CAD build for the part. Positions are in the model's coordinates, mm. A direction names the side the tool comes from. Give positions to 0.01 mm unless a question says otherwise; leave off trailing zeros. Order: outer loops, then holes, each group sorted by start corner. A loop starts at its lowest first (then second) coordinate and runs counter-clockwise, first axis right, second up. Notation, with made-up numbers: M -29.75,18 L -7.75,18 A24 cw -7.75,52 Z; hole C -17.5,27.25 d2. An arc over 180 degrees is marked long. Put each result on its own line as item: value. Start each with the question number.
1) Cut at B-B (y = 21.5). Write the cut outline in (x, z) (3 decimals).
2) Cut at C-C (x = 14). Write the cut outline in (y, z) (3 decimals).
3) Cut at A-A (x = 37). Write the cut outline in (y, z) (3 decimals), and give its area (3 significant figures).
4) Tool access for faces 4 (the face through (46, -3.048, 2)), 5 (the face through (-7, 71.843, 2)), 6 (the face through (61.722, 83, 2)): list every direction of +Z, -Z, +X, -X, +Y, -Y with a clear straight run to the whole face (end or side of a thin tool).
5) Two-plate mould, pull along X, no slides. Class faces 1 (the face through (64, -3.048, 2)), 2 (the face through (-4.824, 88.582, 1.565)), 3 (the face through (10, -3.048, 2)): released by +X, released by -X, zero draft, split by the parting line, or undercut.
6) Drill centre lines: line 1 (X direction, y = 49, z = 2.4); line 2 (Y direction, x = 3.5, z = 0.4); line 3 (Y direction, x = 14, z = 0.55). Where is each one in solid material? Low to high. Write a range as [from, to].
7) Cut at D-D (z = 0.65). Give the number of separate pieces and of enclosed holes in the cut face, and give its area (3 significant figures).
8) Pin check, flat tips, straight feed: pin 1 (1.6 mm diameter, centred on y = 41, z = 1.5, fed in from +X); pin 2 (1.6 mm diameter, centred on x = 63.5, z = 1, fed in from +Y); pin 3 (0.9 mm diameter, centred on y = -2, z = 1, fed in from +X); pin 4 (3 mm diameter, centred on x = 65.41, y = 75.53, fed in from +Z). Stop position of each tip, or through.
```python
from build123d import *

# Parameters (mm, degrees)
SKETCH1_W           = 12.7
SKETCH1_H           = 3.048
SKETCH1_R           = 1.397
SKETCH1_W_2         = 48.514
SKETCH1_H_2         = 1.8034
BOSS_EXTRUDE1_DEPTH = 3.175
SKETCH6_W           = 48.514
SKETCH6_H           = 3.048
CUT_EXTRUDE2_DEPTH  = 4.175
SKETCH5_R           = 3.6891
SKETCH5_R_2         = 2
BOSS_EXTRUDE3_DEPTH = 3.175


with BuildPart() as part:
    # Sketch1 → Boss-Extrude1 (new body)
    with BuildSketch(Plane.XY):
        with BuildLine():
            Line((38.227, 7.112), (38.227, 0))
            Line((38.227, 0), (38.227, -5.588))
            Line((38.227, -5.588), (59.182, -5.588))
            ThreePointArc((59.182, -5.588), (60.978051224, -4.844051224), (61.722, -3.048))
            Line((61.722, -3.048), (61.722, 86.7664))
            ThreePointArc((61.722, 86.7664), (60.978051224, 88.562451224), (59.182, 89.3064))
            Line((59.182, 89.3064), (-3.048, 89.3064))
            ThreePointArc((-3.048, 89.3064), (-4.844051224, 88.562451224), (-5.588, 86.7664))
            Line((-5.588, 86.7664), (-5.588, -3.048))
            ThreePointArc((-5.588, -3.048), (-4.844051224, -4.844051224), (-3.048, -5.588))
            Line((-3.048, -5.588), (22.9616, -5.588))
            Line((22.9616, -5.588), (22.9616, 0))
            Line((22.9616, 0), (22.9616, 7.112))
            Line((22.9616, 7.112), (38.227, 7.112))
        make_face()
        with Locations((9.652, -1.524)):
            Rectangle(SKETCH1_W, SKETCH1_H, mode=Mode.SUBTRACT)
        with Locations((3.556, 3.556)):
            Circle(SKETCH1_R, mode=Mode.SUBTRACT)
        with Locations((46.482, -1.524)):
            Rectangle(SKETCH1_W, SKETCH1_H, mode=Mode.SUBTRACT)
        with Locations((52.578, 3.556)):
            Circle(SKETCH1_R, mode=Mode.SUBTRACT)
        Polygon((-3.048, 6.35), (-3.048, 78.613), (0, 78.613), (0, 61.595), (0, 6.35), align=None, mode=Mode.SUBTRACT)
        with Locations((3.556, 61.595)):
            Circle(SKETCH1_R, mode=Mode.SUBTRACT)
        with Locations((28.067, 85.8647)):
            Rectangle(SKETCH1_W_2, SKETCH1_H_2, mode=Mode.SUBTRACT)
        Polygon((56.134, 78.613), (59.182, 78.613), (59.182, 6.35), (56.134, 6.35), (56.134, 61.595), align=None, mode=Mode.SUBTRACT)
        with Locations((52.578, 61.595)):
            Circle(SKETCH1_R, mode=Mode.SUBTRACT)
    extrude(amount=BOSS_EXTRUDE1_DEPTH)

    # Sketch6 → Cut-Extrude2 (cut, through all)
    with BuildSketch(Plane.XY.offset(3.175)):
        with Locations((28.067, 86.487)):
            Rectangle(SKETCH6_W, SKETCH6_H)
    extrude(amount=-CUT_EXTRUDE2_DEPTH, mode=Mode.SUBTRACT)

    # Sketch5 → Boss-Extrude3 (add)
    with BuildSketch(Plane.XY.offset(3.175)):
        with BuildLine():
            Line((-5.588, 4.3302), (-9.2771, 4.3302))
            ThreePointArc((-9.2771, 4.3302), (-6.668512374, 3.249687626), (-5.588, 0.6411))
            Line((-5.588, 0.6411), (-5.588, 4.3302))
        make_face()
        with BuildLine():
            Line((-5.588, -3.048), (-5.588, 0.6411))
            ThreePointArc((-5.588, 0.6411), (-6.668512374, -1.967487626), (-9.2771, -3.048))
            Line((-9.2771, -3.048), (-5.588, -3.048))
        make_face()
        with Locations((-9.2771, 0.6411)):
            Circle(SKETCH5_R)
        with Locations((-9.2771, 0.6411)):
            Circle(SKETCH5_R_2, mode=Mode.SUBTRACT)
        with Locations((65.4111, 0.6411)):
            Circle(SKETCH5_R)
        with Locations((65.4111, 0.6411)):
            Circle(SKETCH5_R_2, mode=Mode.SUBTRACT)
        with BuildLine():
            Line((61.722, -3.048), (65.4111, -3.048))
            ThreePointArc((65.4111, -3.048), (62.802512374, -1.967487626), (61.722, 0.6411))
            Line((61.722, 0.6411), (61.722, -3.048))
        make_face()
        with BuildLine():
            Line((61.722, 4.3302), (61.722, 0.6411))
            ThreePointArc((61.722, 0.6411), (62.802512374, 3.249687626), (65.4111, 4.3302))
            Line((65.4111, 4.3302), (61.722, 4.3302))
        make_face()
        with Locations((65.4111, 75.5325)):
            Circle(SKETCH5_R)
        with Locations((65.4111, 75.5325)):
            Circle(SKETCH5_R_2, mode=Mode.SUBTRACT)
        with BuildLine():
            Line((61.722, 71.8434), (65.4111, 71.8434))
            ThreePointArc((65.4111, 71.8434), (62.802512374, 72.923912374), (61.722, 75.5325))
            Line((61.722, 75.5325), (61.722, 71.8434))
        make_face()
        with BuildLine():
            Line((61.722, 79.2216), (61.722, 75.5325))
            ThreePointArc((61.722, 75.5325), (62.802512374, 78.141087626), (65.4111, 79.2216))
            Line((65.4111, 79.2216), (61.722, 79.2216))
        make_face()
        with BuildLine():
            Line((-5.588, 71.8434), (-5.588, 75.5325))
            ThreePointArc((-5.588, 75.5325), (-6.668512374, 72.923912374), (-9.2771, 71.8434))
            Line((-9.2771, 71.8434), (-5.588, 71.8434))
        make_face()
        with Locations((-9.2771, 75.5325)):
            Circle(SKETCH5_R)
        with Locations((-9.2771, 75.5325)):
            Circle(SKETCH5_R_2, mode=Mode.SUBTRACT)
        with BuildLine():
            Line((-5.588, 79.2216), (-9.2771, 79.2216))
            ThreePointArc((-9.2771, 79.2216), (-6.668512374, 78.141087626), (-5.588, 75.5325))
            Line((-5.588, 75.5325), (-5.588, 79.2216))
        make_face()
    extrude(amount=-BOSS_EXTRUDE3_DEPTH)


solid = part.part
```
Solution:
1. outline: M -5.588,0 L -3.048,0 L -3.048,3.175 L -5.588,3.175 Z; M 0,0 L 56.134,0 L 56.134,3.175 L 0,3.175 Z; M 59.182,0 L 61.722,0 L 61.722,3.175 L 59.182,3.175 Z
2. outline: M -5.588,0 L -3.048,0 L -3.048,3.175 L -5.588,3.175 Z; M 0,0 L 84.963,0 L 84.963,3.175 L 0,3.175 Z; M 88.011,0 L 89.306,0 L 89.306,3.175 L 88.011,3.175 Z
3. outline: M 7.112,0 L 84.963,0 L 84.963,3.175 L 7.112,3.175 Z; M 88.011,0 L 89.306,0 L 89.306,3.175 L 88.011,3.175 Z
3. area: 251 mm²
4. face 4: +Z, -Z
4. face 5: +Z, -Z, -X
4. face 6: +Z, -Z, +X, +Y
5. face 1: zero draft
5. face 2: released by -X
5. face 3: undercut
6. line 1: [-5.59, -3.05], [0, 56.13], [59.18, 61.72]
6. line 2: [-5.59, -3.05], [0, 2.16], [4.95, 60.2], [62.99, 89.31]
6. line 3: [-5.59, -3.05], [0, 84.96], [88.01, 89.31]
7. separate pieces: 1
7. enclosed holes: 13
7. area: 5,640 mm²
8. pin 1: x = 61.72
8. pin 2: y = 79.22
8. pin 3: x = 68.38
8. pin 4: through
